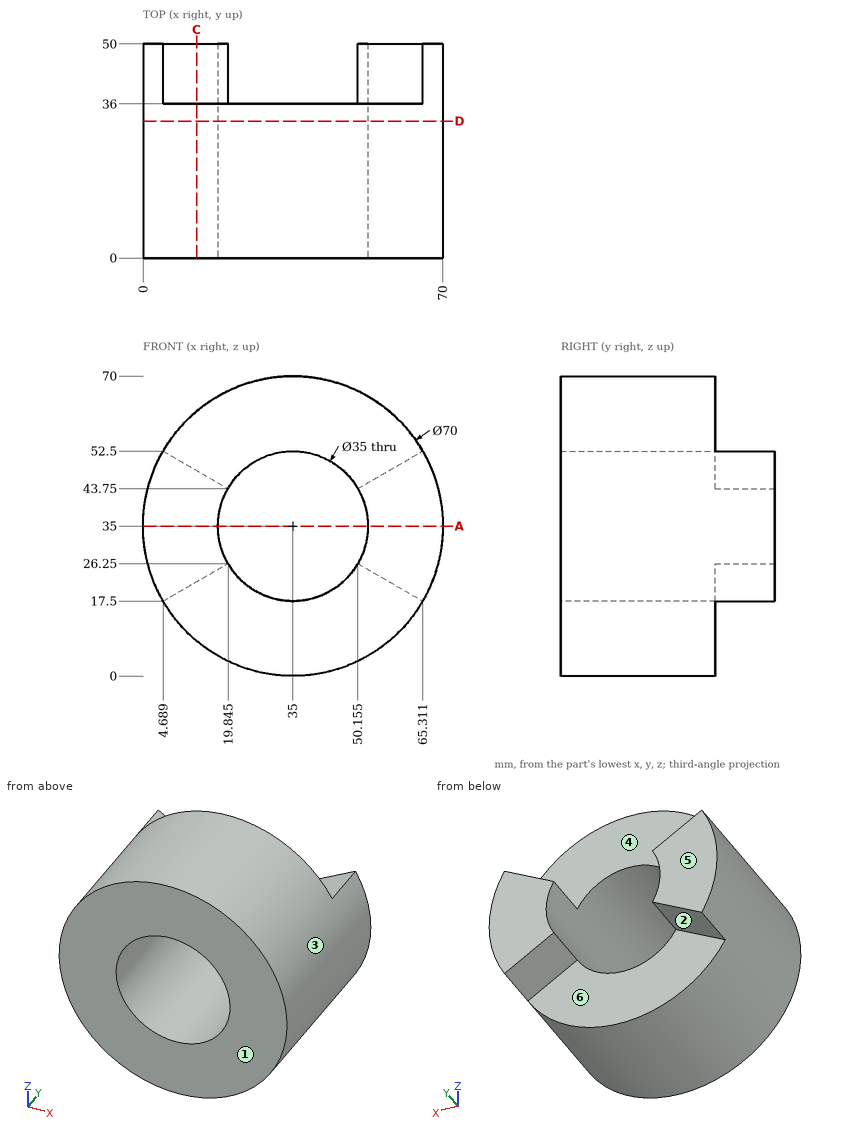
The drawing under review shows one solid part. Ordinate dimensions are in mm from its lowest x, y, z. A direction names the side the tool comes from. Give positions to 0.01 mm unless a question says otherwise; leave off trailing zeros. Order: outer loops, then holes, each group sorted by start corner. A loop starts at its lowest first (then second) coordinate and runs counter-clockwise, first axis right, second up. Notation, with made-up numbers: M -29.75,-7 L 17.25,-7 A21 ccw 17.25,13 Z; hole C -25.75,-24 d9. An arc over 180 degrees is marked long. Answer in a Markdown table with one row per item. Add a question column.
1. Machinability: for the marked faces 4, 5 and 6, which of the approach directions +Z, -Z, +X, -X, +Y, -Y give a long, thin tool a straight path to every point of the face, cutting with its end or side? Answer none if there is none.
2. Add section C-C on x = 12.5. State the section outline as (y, z) points.
3. To check wall thickness, follow line 1 along X through (y, z) = (14, 35); line 2 along Y through (x, z) = (19, 10); line 3 along Z through (x, y) = (42, 30). State the ranges of each line that lie inside material, in increasing order.
4. Add section D-D on y = 32. State the section outline as (x, z) points.
5. Mouldability with a two-part tool opening along X and no side actions: class the marked faces 1, 2 and 3 as released by +X, released by -X, zero draft, split by the parting line, or undercut.
6. Add section A-A on z = 35. State the section outline as (x, y) points, plus the area to 3 significant figures.
7. For pin 1 Ø1 at (x, y) = (43, 5.5) entering from -Z; pin 2 Ø21 at (x, z) = (43.5, 6.5) entering from +Y; pin 3 Ø2 at (y, z) = (20, 18) entering from -X; pin 4 Ø1.5 at (x, z) = (62, 14.5) entering from -Y, all flat-tipped, find the tip position at first contact; note any pin that passes through.
The answers:
| question | item | result |
|---|---|---|
| 1 | face 4 | +Z, +Y |
| 1 | face 5 | +Z, -Z, +X, -X, +Y |
| 1 | face 6 | -Z, +Y |
| 2 | outline | M 0,8.19 L 36,8.19 L 36,22.01 L 50,22.01 L 50,47.99 L 36,47.99 L 36,61.81 L 0,61.81 Z |
| 3 | line 1 | 0 to 17.5, 52.5 to 70 |
| 3 | line 2 | 0 to 36 |
| 3 | line 3 | 0.71 to 18.96, 51.04 to 69.29 |
| 4 | outline | C 35,35 d70; hole C 35,35 d35 |
| 5 | face 1 | zero draft |
| 5 | face 2 | undercut |
| 5 | face 3 | split by the parting line |
| 6 | outline | M 0,0 L 17.5,0 L 17.5,50 L 0,50 Z; M 52.5,0 L 70,0 L 70,50 L 52.5,50 Z |
| 6 | area | 1,750 mm2 |
| 7 | pin 1 | z = 0.81 |
| 7 | pin 2 | y = 36 |
| 7 | pin 3 | x = 3.87 |
| 7 | pin 4 | y = 0 |
